Could you check a few things on this drawing? It's one solid part, dimensions in mm from its lowest x, y, z. A direction names the side the tool comes from. Give positions to 0.01 mm unless a question says otherwise; leave off trailing zeros. Write each loop counter-clockwise with the first axis right and the second up, starting at its lowest first coordinate (ties: lowest second). Pieces come first, ordered by that corner, then holes. Notation, with made-up numbers: (-38, 81.25) - (12, 81.25) arc R30 ccw to (12, 108.25) - close; hole circle Ø8 at (-12, 28.5). An arc over 180 degrees is marked (long way). One line per item, written item: value. Start each with the question number.
1) On a 3-axis mill with a long thin cutter (end or side, diameter ignored), from which of +Z, -Z, +X, -X, +Y, -Y can I reach the whole of each face in a straight line? I mean the marked faces 1 and 2. Say none if no direction works.
2) I'm going to push flat-ended pins straight in: P1, Ø3, axis at x = 12.5, z = 4, coming from the +Y side; P2, Ø6, axis at x = 37, z = 10, coming from the +Y side; P3, Ø10.5, axis at x = 24, z = 8.5, coming from the +Y side. Where does each tip first touch, or does it pass through?
3) We'd pull the mould along X, two halves only. Please class the marked faces 3, 4 and 5: +X half, -X half, draft (parallel to the pull), parting line (faces both ways), or undercut.
4) Imagine slicing it at D-D on x = 46.5. Write out the boundary of the cut face in (y, z), plus the area to 3 significant figures.
5) Imagine slicing it at C-C on y = 20. Write out the boundary of the cut face in (x, z).
6) Imagine slicing it at A-A on z = 10.16. Write out the boundary of the cut face in (x, y).
7) Please list where these lines run through material, in increasing order: L1, parallel to X at y = 15.5, z = 1.75; L2, parallel to Z at x = 10, y = 25. Write a range as [from, to].
8) Imagine slicing it at B-B on x = 12.7. Write out the boundary of the cut face in (y, z).
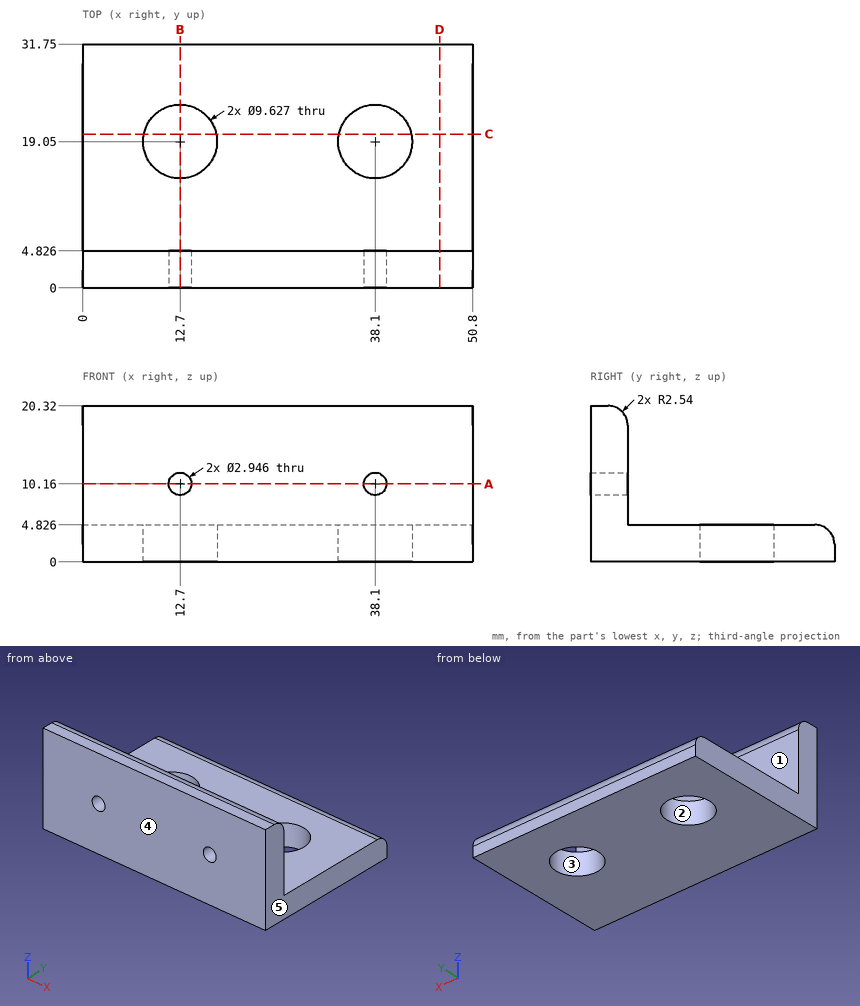
Numbers:
1. face 1: +Z, +X, -X, +Y
1. face 2: +Z, -Z
2. P1: y = 31.74
2. P2: y = 4.83
2. P3: y = 31.56
3. face 3: undercut
3. face 4: draft
3. face 5: +X half
4. outline: (0, 0) - (31.75, 0) - (31.75, 2.29) arc R2.54 ccw to (29.21, 4.83) - (4.83, 4.83) - (4.83, 17.78) arc R2.54 ccw to (2.29, 20.32) - (0, 20.32) - close
4. area: 225 mm^2
5. outline: (0, 0) - (7.98, 0) - (7.98, 4.83) - (0, 4.83) - close; (17.42, 0) - (33.38, 0) - (33.38, 4.83) - (17.42, 4.83) - close; (42.82, 0) - (50.8, 0) - (50.8, 4.83) - (42.82, 4.83) - close
6. outline: (0, 0) - (11.23, 0) - (11.23, 4.83) - (0, 4.83) - close; (14.17, 0) - (36.63, 0) - (36.63, 4.83) - (14.17, 4.83) - close; (39.57, 0) - (50.8, 0) - (50.8, 4.83) - (39.57, 4.83) - close
7. L1: [0, 9.45], [15.95, 34.85], [41.35, 50.8]
7. L2: [0, 4.83]
8. outline: (0, 0) - (14.24, 0) - (14.24, 4.83) - (4.83, 4.83) - (4.83, 8.69) - (0, 8.69) - close; (0, 11.63) - (4.83, 11.63) - (4.83, 17.78) arc R2.54 ccw to (2.29, 20.32) - (0, 20.32) - close; (23.86, 0) - (31.75, 0) - (31.75, 2.29) arc R2.54 ccw to (29.21, 4.83) - (23.86, 4.83) - close
